Source: three-view drawing plus pictorial views. Frame: mm from the lowest corner of the part. A direction names the side the tool comes from. Give positions to 0.01 mm unless a question says otherwise; leave off trailing zeros. Loops run counter-clockwise (first coordinate to the right, second up) from the corner with the lowest first, then second, coordinate; pieces in that order, holes last.
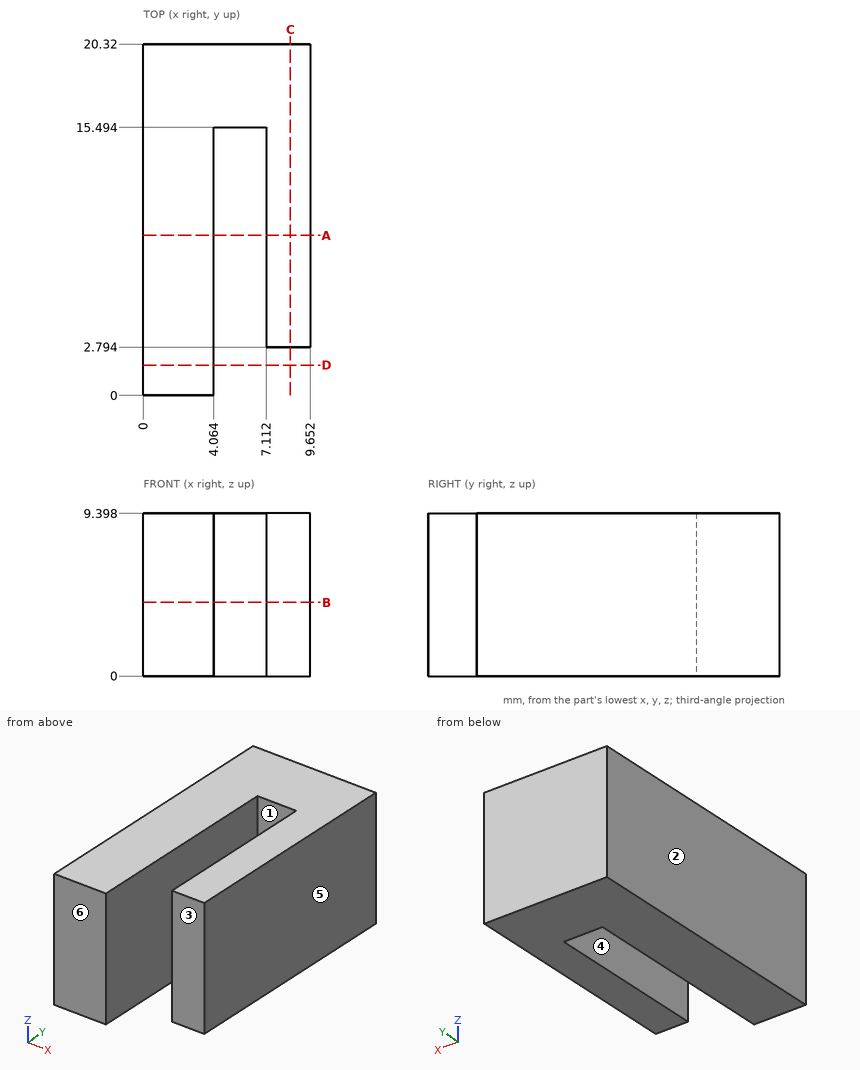
Q1. Section query A-A, the plane y = 9.25. Return loops of the section in (x, z), and give its area (3 significant figures).
Q2. Material intervals for probe 1 along X at (y, z) = (12, 5.75); probe 2 along Y at (x, z) = (8.75, 4.75); probe 3 along Y at (x, z) = (4.25, 7), sorted ascending.
Q3. Section query B-B, the plane z = 4.25. Return loops of the section in (x, y).
Q4. Mould query, pull axis X, two halves, no side actions, for the marked faces 4, 5 and 6. Classes: +X half, -X half, draft (parallel to the pull), parting line (faces both ways), or undercut.
Q5. Reachability of the marked faces 1, 2 and 3 from +Z, -Z, +X, -X, +Y, -Y: full face, straight path, thin tool, end or side. Return the list, or none.
Q6. Pin query (flat end, axial travel): pin 1 Ø1.3 at (x, z) = (8.5, 5.5) entering from -Y; pin 2 Ø0.9 at (x, z) = (5.5, 3.5) entering from -Y. Return the tip coordinate at first contact, or that it passes through.
Q7. Section query C-C, the plane x = 8.5. Return loops of the section in (y, z), and give its area (3 significant figures).
Q8. Section query D-D, the plane y = 1.75. Return loops of the section in (x, z), and give its area (3 significant figures).
Resolved:
1. outline: (0, 0) - (4.06, 0) - (4.06, 9.4) - (0, 9.4) - close; (7.11, 0) - (9.65, 0) - (9.65, 9.4) - (7.11, 9.4) - close
1. area: 62.1 mm2
2. probe 1: x = 0 to 4.06, 7.11 to 9.65
2. probe 2: y = 2.79 to 20.32
2. probe 3: y = 15.49 to 20.32
3. outline: (0, 0) - (4.06, 0) - (4.06, 15.49) - (7.11, 15.49) - (7.11, 2.79) - (9.65, 2.79) - (9.65, 20.32) - (0, 20.32) - close
4. face 4: undercut
4. face 5: +X half
4. face 6: draft
5. face 1: +Z, -Z, -Y
5. face 2: +Z, -Z, -X, +Y, -Y
5. face 3: +Z, -Z, +X, -Y
6. pin 1: stops at y = 2.79
6. pin 2: stops at y = 15.49
7. outline: (2.79, 0) - (20.32, 0) - (20.32, 9.4) - (2.79, 9.4) - close
7. area: 165 mm2
8. outline: (0, 0) - (4.06, 0) - (4.06, 9.4) - (0, 9.4) - close
8. area: 38.2 mm2
